from build123d import *

# Parameters (mm, degrees)
SKETCH1_R               = 1.5
BOSS_EXTRUDE1_DEPTH     = 2
BOSS_EXTRUDE3_DEPTH     = 8
FILLET2_R               = 1
SKETCH6_R               = 1.5
SKETCH6_W               = 3
SKETCH6_H               = 15
BOSS_EXTRUDE5_DEPTH     = 6
FILLET3_R               = 2
SKETCH7_R               = 1.5
CUT_EXTRUDE1_DEPTH      = 51
CUT_EXTRUDE1_DEPTH_BACK = 51
SKETCH8_R               = 1.5
CUT_EXTRUDE2_DEPTH      = 51
CUT_EXTRUDE2_DEPTH_BACK = 51


with BuildPart() as part:
    # Sketch1 → Boss-Extrude1 (new body)
    with BuildSketch(Plane.XY):
        with BuildLine():
            Line((-50, 40), (-48, 40))
            Line((-48, 40), (-48, 25))
            Line((-48, 25), (-50, 25))
            Line((-50, 25), (-50, -25))
            Line((-50, -25), (-48, -25))
            Line((-48, -25), (-48, -40))
            Line((-48, -40), (-50, -40))
            Line((-50, -40), (-50, -49))
            ThreePointArc((-50, -49), (-49.707106781, -49.707106781), (-49, -50))
            Line((-49, -50), (-40, -50))
            Line((-40, -50), (-40, -48))
            Line((-40, -48), (-25, -48))
            Line((-25, -48), (-25, -50))
            Line((-25, -50), (25, -50))
            Line((25, -50), (25, -48))
            Line((25, -48), (40, -48))
            Line((40, -48), (40, -50))
            Line((40, -50), (49, -50))
            ThreePointArc((49, -50), (49.707106781, -49.707106781), (50, -49))
            Line((50, -49), (50, -40))
            Line((50, -40), (48, -40))
            Line((48, -40), (48, -25))
            Line((48, -25), (50, -25))
            Line((50, -25), (50, 25))
            Line((50, 25), (48, 25))
            Line((48, 25), (48, 40))
            Line((48, 40), (50, 40))
            Line((50, 40), (50, 49))
            ThreePointArc((50, 49), (49.707106781, 49.707106781), (49, 50))
            Line((49, 50), (40, 50))
            Line((40, 50), (40, 48))
            Line((40, 48), (25, 48))
            Line((25, 48), (25, 50))
            Line((25, 50), (-25, 50))
            Line((-25, 50), (-25, 48))
            Line((-25, 48), (-40, 48))
            Line((-40, 48), (-40, 50))
            Line((-40, 50), (-49, 50))
            ThreePointArc((-49, 50), (-49.707106781, 49.707106781), (-50, 49))
            Line((-50, 49), (-50, 40))
        make_face()
        with Locations((-45, 22)):
            Circle(SKETCH1_R, mode=Mode.SUBTRACT)
        with Locations((-22, 45)):
            Circle(SKETCH1_R, mode=Mode.SUBTRACT)
        with Locations((22, 45)):
            Circle(SKETCH1_R, mode=Mode.SUBTRACT)
        with Locations((45, 22)):
            Circle(SKETCH1_R, mode=Mode.SUBTRACT)
        with Locations((45, -22)):
            Circle(SKETCH1_R, mode=Mode.SUBTRACT)
        with Locations((22, -45)):
            Circle(SKETCH1_R, mode=Mode.SUBTRACT)
        with Locations((-22, -45)):
            Circle(SKETCH1_R, mode=Mode.SUBTRACT)
        with Locations((-45, -22)):
            Circle(SKETCH1_R, mode=Mode.SUBTRACT)
        with BuildLine():
            Line((-30, -40), (30, -40))
            ThreePointArc((30, -40), (37.071067812, -37.071067812), (40, -30))
            Line((40, -30), (40, 30))
            ThreePointArc((40, 30), (37.071067812, 37.071067812), (30, 40))
            Line((30, 40), (-30, 40))
            ThreePointArc((-30, 40), (-37.071067812, 37.071067812), (-40, 30))
            Line((-40, 30), (-40, -30))
            ThreePointArc((-40, -30), (-37.071067812, -37.071067812), (-30, -40))
        make_face(mode=Mode.SUBTRACT)
    extrude(amount=BOSS_EXTRUDE1_DEPTH)

    # Sketch2 → Boss-Extrude3 (add)
    with BuildSketch(Plane.XY.offset(2)):
        with BuildLine():
            Line((-49, 50), (-40, 50))
            Line((-40, 50), (-40, 40))
            Line((-40, 40), (-50, 40))
            Line((-50, 40), (-50, 49))
            ThreePointArc((-50, 49), (-49.707106781, 49.707106781), (-49, 50))
        make_face()
        with BuildLine():
            Line((40, 50), (40, 40))
            Line((40, 40), (50, 40))
            Line((50, 40), (50, 49))
            ThreePointArc((50, 49), (49.707106781, 49.707106781), (49, 50))
            Line((49, 50), (40, 50))
        make_face()
        with BuildLine():
            Line((49, -50), (40, -50))
            Line((40, -50), (40, -40))
            Line((40, -40), (50, -40))
            Line((50, -40), (50, -49))
            ThreePointArc((50, -49), (49.707106781, -49.707106781), (49, -50))
        make_face()
        with BuildLine():
            Line((-40, -50), (-40, -40))
            Line((-40, -40), (-50, -40))
            Line((-50, -40), (-50, -49))
            ThreePointArc((-50, -49), (-49.707106781, -49.707106781), (-49, -50))
            Line((-49, -50), (-40, -50))
        make_face()
    extrude(amount=BOSS_EXTRUDE3_DEPTH)

    # Fillet2
    fillet2_edges = [part.edges().sort_by_distance(p)[0] for p in [
        (-40, 40, 6),
        (-40, 45, 10),
        (-44.5, 50, 10),
        (-49.707106781, 49.707106781, 10),
        (-50, 44.5, 10),
        (-45, 40, 10),
        (40, 40, 6),
        (50, 44.5, 10),
        (49.707106781, 49.707106781, 10),
        (44.5, 50, 10),
        (40, 45, 10),
        (45, 40, 10),
        (40, -40, 6),
        (40, -45, 10),
        (44.5, -50, 10),
        (49.707106781, -49.707106781, 10),
        (50, -44.5, 10),
        (45, -40, 10),
        (-40, -40, 6),
        (-50, -44.5, 10),
        (-49.707106781, -49.707106781, 10),
        (-44.5, -50, 10),
        (-40, -45, 10),
        (-45, -40, 10),
        (-50, -40, 5),
        (-50, 40, 5),
        (-40, 50, 5),
        (40, 50, 5),
        (50, 40, 5),
        (50, -40, 5),
        (40, -50, 5),
        (-40, -50, 5),
    ]]
    fillet(fillet2_edges, radius=FILLET2_R)

    # Sketch6 → Boss-Extrude5 (add)
    with BuildSketch(Plane(origin=(0, 0, 0), x_dir=(-1, 0, 0), z_dir=(0, 0, -1))):
        with BuildLine():
            Line((-43, 48), (-43, 42.85))
            ThreePointArc((-43, 42.85), (-40, 39.85), (-37, 42.85))
            Line((-37, 42.85), (-37, 44))
            ThreePointArc((-37, 44), (-36.707106781, 44.707106781), (-36, 45))
            Line((-36, 45), (-25, 45))
            Line((-25, 45), (-25, 48))
            Line((-25, 48), (-43, 48))
        make_face()
        with Locations((-40, 42.85)):
            Circle(SKETCH6_R, mode=Mode.SUBTRACT)
        with BuildLine():
            Line((25, 48), (25, 45))
            Line((25, 45), (36, 45))
            ThreePointArc((36, 45), (36.707106781, 44.707106781), (37, 44))
            Line((37, 44), (37, 42.85))
            ThreePointArc((37, 42.85), (40, 39.85), (43, 42.85))
            Line((43, 42.85), (43, 48))
            Line((43, 48), (25, 48))
        make_face()
        with Locations((40, 42.85)):
            Circle(SKETCH6_R, mode=Mode.SUBTRACT)
        with BuildLine():
            Line((-40.4, -48), (-40.4, -42.85))
            ThreePointArc((-40.4, -42.85), (-37.4, -39.85), (-34.4, -42.85))
            Line((-34.4, -42.85), (-34.4, -44))
            ThreePointArc((-34.4, -44), (-34.107106781, -44.707106781), (-33.4, -45))
            Line((-33.4, -45), (-25, -45))
            Line((-25, -45), (-25, -48))
            Line((-25, -48), (-40.4, -48))
        make_face()
        with Locations((-37.4, -42.85)):
            Circle(SKETCH6_R, mode=Mode.SUBTRACT)
        with BuildLine():
            Line((25, -48), (25, -45))
            Line((25, -45), (32.2, -45))
            ThreePointArc((32.2, -45), (32.907106781, -44.707106781), (33.2, -44))
            Line((33.2, -44), (33.2, -42.85))
            ThreePointArc((33.2, -42.85), (36.2, -39.85), (39.2, -42.85))
            Line((39.2, -42.85), (39.2, -48))
            Line((39.2, -48), (25, -48))
        make_face()
        with Locations((36.2, -42.85)):
            Circle(SKETCH6_R, mode=Mode.SUBTRACT)
        with Locations((-46.5, 32.5)):
            Rectangle(SKETCH6_W, SKETCH6_H)
        with Locations((46.5, 32.5)):
            Rectangle(SKETCH6_W, SKETCH6_H)
        with Locations((-46.5, -32.5)):
            Rectangle(SKETCH6_W, SKETCH6_H)
        with Locations((46.5, -32.5)):
            Rectangle(SKETCH6_W, SKETCH6_H)
    extrude(amount=BOSS_EXTRUDE5_DEPTH)

    # Fillet3
    fillet3_edges = [part.edges().sort_by_distance(p)[0] for p in [
        (25, 46.5, -6),
        (-25, 46.5, -6),
        (25, -46.5, -6),
        (-25, -46.5, -6),
        (46.5, 25, -6),
        (46.5, 40, -6),
        (-46.5, 40, -6),
        (-46.5, 25, -6),
        (46.5, -40, -6),
        (46.5, -25, -6),
        (-46.5, -25, -6),
        (-46.5, -40, -6),
    ]]
    fillet(fillet3_edges, radius=FILLET3_R)

    # Sketch7 → Cut-Extrude1 (cut, two sides)
    with BuildSketch(Plane(origin=(0, 0, 0), x_dir=(0, 0, -1), z_dir=(1, 0, 0))) as cut_extrude1_sk:
        with Locations((2.5, 35.5)):
            Circle(SKETCH7_R)
        with Locations((2.5, 29.5)):
            Circle(SKETCH7_R)
        with Locations((2.5, -29.5)):
            Circle(SKETCH7_R)
        with Locations((2.5, -35.5)):
            Circle(SKETCH7_R)
    extrude(amount=CUT_EXTRUDE1_DEPTH, mode=Mode.SUBTRACT)
    extrude(cut_extrude1_sk.sketch, amount=-CUT_EXTRUDE1_DEPTH_BACK, mode=Mode.SUBTRACT)

    # Sketch8 → Cut-Extrude2 (cut, two sides)
    with BuildSketch(Plane(origin=(0, 0, 0), x_dir=(1, 0, 0), z_dir=(0, 1, 0))) as cut_extrude2_sk:
        with Locations((-29.5, 2.5)):
            Circle(SKETCH8_R)
        with Locations((29.5, 2.5)):
            Circle(SKETCH8_R)
    extrude(amount=CUT_EXTRUDE2_DEPTH, mode=Mode.SUBTRACT)
    extrude(cut_extrude2_sk.sketch, amount=-CUT_EXTRUDE2_DEPTH_BACK, mode=Mode.SUBTRACT)


solid = part.part
Input: part model. Units: mm. Frame: model coordinates. A direction names the side the tool comes from. Give positions to 0.01 mm unless a question says otherwise; leave off trailing zeros. Write each loop counter-clockwise with the first axis right and the second up, starting at its lowest first coordinate (ties: lowest second). Pieces come first, ordered by that corner, then holes. Notation, with made-up numbers: M 85,-16 L 119,-16 A33 ccw 119,21 Z; hole C 32,18 d7. An arc over 180 degrees is marked long. Write item = value, one per line. Start each with the question number.
1) Cut plane A-A on y = -17. Return the cut outline in (x, z).
2) Draft query along X for faces 4 (the flat face through (-48, -32, -2)), 5 (the flat face through (-36, -43, 0)), 6 (the flat face through (45, -50, 4)). Return one class per face: +X half, -X half, draft (parallel to the pull), parting line (faces both ways), or undercut.
3) First-contact query: pin 1 Ø3.5 at (x, z) = (46, -2.5) entering from +Y; pin 2 Ø1.5 at (x, z) = (-46, -2.5) entering from -Y; pin 3 Ø3.5 at (y, z) = (-46.5, -2) entering from +X; pin 4 Ø6 at (x, z) = (30, 7.5) entering from -Y. Flat tips, straight axial feed; report the tip coordinate or a pass-through.
4) Reachability of faces 1 (the flat face through (0, -41, 2)), 2 (the cylindrical face through (-36.13, -39.85, -2.96)), 3 (the flat face through (47, -40, -2)) from +Z, -Z, +X, -X, +Y, -Y: full face, straight path, thin tool, end or side. Return the list, or none.
5) Material intervals for line 1 along X through (y, z) = (-45.95, -2.5); line 2 along Y through (x, z) = (46.95, -2.5); line 3 along Y through (x, z) = (-36.2, -2.7), sorted ascending. Write a range as [from, to].
6) Cut plane C-C on z = 4.5. Count the separate pieces of the cut face and the enclosed holes in it, then the cut area to 3 significant figures.
Solved:
q1.outline = M -50,0 L -40,0 L -40,2 L -50,2 Z; M 40,0 L 50,0 L 50,2 L 40,2 Z
q2.face_4 = -X half
q2.face_5 = undercut
q2.face_6 = draft
q3.pin_1 = 40
q3.pin_2 = -40
q3.pin_3 = 40.4
q3.pin_4 = through
q4.face_1 = +Z
q4.face_2 = -Z
q4.face_3 = -Z, +X, -Y
q5.line_1 = [-39.2, -31], [-28, -25], [25, 28], [31, 40.4]
q5.line_2 = [-40, -37], [-34, -31], [-28, -25], [25, 28], [31, 34], [37, 40]
q5.line_3 = [-48, -44.35], [-41.35, -39.85], [44.98, 48]
q6.separate_pieces = 4
q6.enclosed_holes = 0
q6.area = 397 mm2
